CAD build for the part. Positions are in the model's coordinates, mm. Face numbers are marked on the shaded views. A direction names the side the tool comes from. Round coordinates to 2 decimals unless told otherwise and drop trailing zeros. Order: outer loops, then holes, each group sorted by start corner. A loop starts at its lowest first (then second) coordinate and runs counter-clockwise, first axis right, second up. Notation, with made-up numbers: (52, 26.5) -> (61, 26.5) arc R20 cw to (61, 50.5) -> close; hole circle Ø6 at (-32.75, -22). An arc over 180 degrees is marked (long way). Answer as CSV lines item,"result". Start each with the question number.
from build123d import *

# Parameters (mm, degrees)
SKETCH_R      = 28
SKETCH_R_2    = 25
PAD_DEPTH     = 7
SKETCH001_R   = 26
SKETCH001_R_2 = 25
PAD001_DEPTH  = 10.5
SKETCH002_R   = 25
PAD002_DEPTH  = 1


with BuildPart() as part:
    # Sketch → Pad (new body)
    with BuildSketch(Plane.XY):
        Circle(SKETCH_R)
        Circle(SKETCH_R_2, mode=Mode.SUBTRACT)
    extrude(amount=PAD_DEPTH)

    # Sketch001 → Pad001 (join)
    with BuildSketch(Plane.XY):
        Circle(SKETCH001_R)
        Circle(SKETCH001_R_2, mode=Mode.SUBTRACT)
    extrude(amount=PAD001_DEPTH)

    # Sketch002 (on DatumPlane) → Pad002 (join)
    with BuildSketch(Plane.XY.offset(9.5)):
        Circle(SKETCH002_R)
        with BuildLine():
            ThreePointArc((-23.473389, -5), (24, 0), (-23.473389, 5))
            ThreePointArc((-23.473389, -5), (-18.473389, 0), (-23.473389, 5))
        make_face(mode=Mode.SUBTRACT)
    extrude(amount=PAD002_DEPTH)


solid = part.part
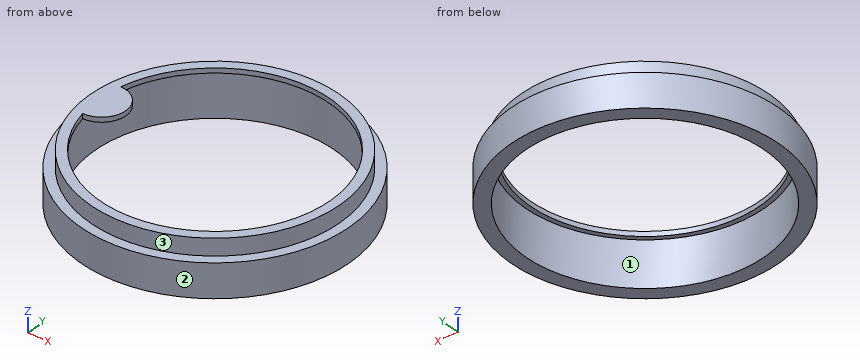
Item 1: Tool access for the marked faces 1, 2 and 3: list every direction of +Z, -Z, +X, -X, +Y, -Y with a clear straight run to the whole face (end or side of a thin tool).
Item 2: Probe line 1 (X direction, y = 0, z = 10.2); line 2 (Z direction, x = -18.5, y = 20); line 3 (Y direction, x = -1.5, z = 3). List the from-to ranges inside material, lowest first.
Item 3: Band-saw the part on B-B, the plane y = 0. Give the cut face in (x, z).
Item 4: Band-saw the part on D-D, the plane x = -21. Give the cut face in (y, z).
Item 5: Band-saw the part on C-C, the plane z = 8. Give the cut face in (x, y).
Item 6: Band-saw the part on A-A, the plane x = 0. Give the cut face in (y, z).
Item 7: Pin check, flat tips, straight feed: pin 1 (5 mm diameter, centred on y = 21, z = 3, fed in from +X); pin 2 (1 mm diameter, centred on y = 5, z = 5, fed in from -X). Stop position of each tip, or through.
Values:
1,face 1,"-Z"
1,face 2,"+Z, -Z"
1,face 3,"+Z"
2,line 1,"-26 to -18.47, 24 to 26"
2,line 2,"0 to 7"
2,line 3,"-27.96 to -24.95, 24.95 to 27.96"
3,outline,"(-28, 0) -> (-25, 0) -> (-25, 9.5) -> (-18.47, 9.5) -> (-18.47, 10.5) -> (-26, 10.5) -> (-26, 7) -> (-28, 7) -> close; (24, 9.5) -> (25, 9.5) -> (25, 0) -> (28, 0) -> (28, 7) -> (26, 7) -> (26, 10.5) -> (24, 10.5) -> close"
4,outline,"(-18.52, 0) -> (-13.56, 0) -> (-13.56, 9.5) -> (-11.62, 9.5) -> (-11.62, 10.5) -> (-15.33, 10.5) -> (-15.33, 7) -> (-18.52, 7) -> close; (-4.35, 9.5) -> (4.35, 9.5) -> (4.35, 10.5) -> (-4.35, 10.5) -> close; (11.62, 9.5) -> (13.56, 9.5) -> (13.56, 0) -> (18.52, 0) -> (18.52, 7) -> (15.33, 7) -> (15.33, 10.5) -> (11.62, 10.5) -> close"
5,outline,"circle Ø52 at (0, 0); hole circle Ø50 at (0, 0)"
6,outline,"(-28, 0) -> (-25, 0) -> (-25, 9.5) -> (-24, 9.5) -> (-24, 10.5) -> (-26, 10.5) -> (-26, 7) -> (-28, 7) -> close; (24, 9.5) -> (25, 9.5) -> (25, 0) -> (28, 0) -> (28, 7) -> (26, 7) -> (26, 10.5) -> (24, 10.5) -> close"
7,pin 1,"x = 21.02"
7,pin 2,"x = -27.64"
